Autodesk Inventor part; units mm, degrees
ref_plane "YZ Plane" through (0, 0, 0) normal (1, 0, 0) x (0, 1, 0)
ref_plane "XZ Plane" through (0, 0, 0) normal (0, 1, 0) x (-1, 0, 0)
ref_plane "XY Plane" through (0, 0, 0) normal (0, 0, 1) x (1, 0, 0)
sketch "Sketch1" plane through (0, 0, 0) normal (0, 0, 1) x (1, 0, 0)
  line L0 (45.72, 0) -> (45.72, 60.96)
  line L1 (45.72, 60.96) -> (-45.72, 60.96)
  line L2 (-45.72, 60.96) -> (-45.72, 9.301)
  line L3 (-45.72, 5.08) -> (-50.8, 5.08)
  line L4 (-50.8, 5.08) -> (-50.8, 15.24)
  line L5 (-50.8, 15.24) -> (-45.72, 15.24)
  line L6 (-45.72, 15.24) -> (-45.72, 5.08)
  line L7 (-45.72, 25.4) -> (-50.8, 25.4)
  line L8 (-50.8, 25.4) -> (-50.8, 35.56)
  line L9 (-50.8, 35.56) -> (-45.72, 35.56)
  line L10 (-45.72, 35.56) -> (-45.72, 25.4)
  line L11 (-45.72, 45.72) -> (-50.8, 45.72)
  line L12 (-50.8, 45.72) -> (-50.8, 55.88)
  line L13 (-50.8, 55.88) -> (-45.72, 55.88)
  line L14 (-45.72, 55.88) -> (-45.72, 45.72)
  line L15 (0, 60.96) -> (0, 0) construction
  line L16 (45.72, 60.96) -> (45.72, 0)
  line L17 (45.72, 5.08) -> (50.8, 5.08)
  line L18 (50.8, 5.08) -> (50.8, 15.24)
  line L19 (50.8, 15.24) -> (45.72, 15.24)
  line L20 (45.72, 15.24) -> (45.72, 5.08)
  line L21 (45.72, 25.4) -> (50.8, 25.4)
  line L22 (50.8, 25.4) -> (50.8, 35.56)
  line L23 (50.8, 35.56) -> (45.72, 35.56)
  line L24 (45.72, 35.56) -> (45.72, 25.4)
  line L25 (45.72, 45.72) -> (50.8, 45.72)
  line L26 (50.8, 45.72) -> (50.8, 55.88)
  line L27 (50.8, 55.88) -> (45.72, 55.88)
  line L28 (45.72, 55.88) -> (45.72, 45.72)
  line L29 (-45.72, 5.08) -> (-45.72, 0)
  line L30 (-45.72, 0) -> (45.72, 0)
  line L31 (45.72, 60.96) -> (-45.72, 60.96)
  line L32 (-45.72, 60.96) -> (-45.72, 0)
  line L33 (-45.72, 0) -> (45.72, 0)
  line L34 (45.72, 0) -> (45.72, 60.96)
  dimension "d0" = 91.44
  dimension "d2" = 10.16
  dimension "d3" = 5.08
  dimension "d7" = 20.32
  dimension "d14" = 5.08
  dimension "d15" = 60.96
extrude "Extrusion2" add sketch "Sketch1" along normal blind 5.08
sketch "Sketch5" plane through (0, 0, 5.08) normal (0, 0, 1) x (1, 0, 0)
  line L0 (50.8, 25.4) -> (50.8, 35.56)
  line L1 (50.8, 35.56) -> (45.72, 35.56)
  line L2 (45.72, 35.56) -> (45.72, 45.72)
  line L3 (45.72, 45.72) -> (50.8, 45.72)
  line L4 (50.8, 45.72) -> (50.8, 55.88)
  line L5 (50.8, 55.88) -> (45.72, 55.88)
  line L6 (45.72, 55.88) -> (45.72, 60.96)
  line L7 (45.72, 60.96) -> (-45.72, 60.96)
  line L8 (-45.72, 60.96) -> (-45.72, 55.88)
  line L9 (-45.72, 55.88) -> (-50.8, 55.88)
  line L10 (-50.8, 55.88) -> (-50.8, 45.72)
  line L11 (-50.8, 45.72) -> (-45.72, 45.72)
  line L12 (-45.72, 45.72) -> (-45.72, 35.56)
  line L13 (-45.72, 35.56) -> (-50.8, 35.56)
  line L14 (-50.8, 35.56) -> (-50.8, 25.4)
  line L15 (-50.8, 25.4) -> (-45.72, 25.4)
  line L16 (-45.72, 25.4) -> (-45.72, 15.24)
  line L17 (-45.72, 15.24) -> (-50.8, 15.24)
  line L18 (-50.8, 15.24) -> (-50.8, 5.08)
  line L19 (-50.8, 5.08) -> (-45.72, 5.08)
  line L20 (-45.72, 5.08) -> (-45.72, 0)
  line L21 (-45.72, 0) -> (45.72, 0)
  line L22 (45.72, 0) -> (45.72, 5.08)
  line L23 (45.72, 5.08) -> (50.8, 5.08)
  line L24 (50.8, 5.08) -> (50.8, 15.24)
  line L25 (50.8, 15.24) -> (45.72, 15.24)
  line L26 (45.72, 15.24) -> (45.72, 25.4)
  line L27 (45.72, 25.4) -> (50.8, 25.4)
  line L28 (-24.13, 30.48) -> (24.13, 30.48) construction
  line L29 (-24.13, 21.59) -> (24.13, 21.59)
  line L30 (24.13, 39.37) -> (-24.13, 39.37)
  arc A0 (-24.13, 39.37) -> (-24.13, 21.59) centre (-24.13, 30.48) ccw
  arc A1 (24.13, 21.59) -> (24.13, 39.37) centre (24.13, 30.48) ccw
  line L31 (45.72, 60.96) -> (-45.72, 60.96) construction
  line L32 (0, 60.96) -> (0, 0) construction
  point P0 (0, 30.48)
  dimension "d32" = 48.26
  dimension "d33" = 60.96
  dimension "d34" = 30.48
  dimension "d35" = 8.89
extrude "Extrusion6" cut sketch "Sketch5" against normal blind 25.4 contours A0 L30 A1 L29
sketch "Sketch6" plane through (0, 0, 0) normal (0, 0, -1) x (-1, 0, 0)
  arc A0 (-24.13, 39.37) -> (-24.13, 21.59) centre (-24.13, 30.48) ccw
  line L0 (-24.13, 39.37) -> (24.13, 39.37)
  arc A1 (24.13, 21.59) -> (24.13, 39.37) centre (24.13, 30.48) ccw
  line L1 (24.13, 21.59) -> (-24.13, 21.59)
  line L2 (-50.8, 35.56) -> (-50.8, 25.4)
  line L3 (-50.8, 25.4) -> (-45.72, 25.4)
  line L4 (-45.72, 15.24) -> (-45.72, 25.4)
  line L5 (-50.8, 15.24) -> (-45.72, 15.24)
  line L6 (-50.8, 5.08) -> (-50.8, 15.24)
  line L7 (-45.72, 5.08) -> (-50.8, 5.08)
  line L8 (-45.72, 0) -> (-45.72, 5.08)
  line L9 (45.72, 0) -> (-45.72, 0) construction
  line L10 (45.72, 5.08) -> (45.72, 0)
  line L11 (50.8, 5.08) -> (45.72, 5.08)
  line L12 (50.8, 15.24) -> (50.8, 5.08)
  line L13 (45.72, 15.24) -> (50.8, 15.24)
  line L14 (45.72, 25.4) -> (45.72, 15.24)
  line L15 (45.72, 25.4) -> (50.8, 25.4)
  line L16 (50.8, 25.4) -> (50.8, 35.56)
  line L17 (50.8, 35.56) -> (45.72, 35.56)
  line L18 (45.72, 45.72) -> (45.72, 35.56)
  line L19 (45.72, 45.72) -> (50.8, 45.72)
  line L20 (50.8, 45.72) -> (50.8, 55.88)
  line L21 (50.8, 55.88) -> (45.72, 55.88)
  line L22 (45.72, 60.96) -> (45.72, 55.88)
  line L23 (-45.72, 60.96) -> (45.72, 60.96)
  line L24 (-45.72, 55.88) -> (-45.72, 60.96)
  line L25 (-50.8, 55.88) -> (-45.72, 55.88)
  line L26 (-50.8, 45.72) -> (-50.8, 55.88)
  line L27 (-45.72, 45.72) -> (-50.8, 45.72)
  line L28 (-45.72, 35.56) -> (-45.72, 45.72)
  line L29 (-45.72, 35.56) -> (-50.8, 35.56)
  line L30 (33.02, 30.48) -> (33.02, 60.96)
  line L31 (-45.72, 60.96) -> (45.72, 60.96)
  arc A2 (-24.13, 39.37) -> (-24.13, 21.59) centre (-24.13, 30.48) ccw
  line L32 (-33.02, 30.48) -> (-33.02, 60.96)
  line L33 (-33.02, 60.96) -> (33.02, 60.96)
  arc A3 (24.13, 21.59) -> (24.13, 39.37) centre (24.13, 30.48) ccw
  line L34 (25.8987, 21.7677) -> (0.6317, 16.6382)
  line L35 (-0.6317, 16.6382) -> (-25.8987, 21.7677)
  arc A4 (24.13, 21.59) -> (24.13, 39.37) centre (24.13, 30.48) ccw
  line L36 (0, 21.59) -> (0, 0) construction
  arc A5 (-0.6317, 16.6382) -> (0.6317, 16.6382) centre (0, 19.7498) ccw
  circle A6 centre (24.13, 30.48) radius 8.89
  circle A7 centre (-24.13, 30.48) radius 8.89
  point P0 (0, 16.51)
  dimension "d38" = 5.08
  dimension "d39" = 3.175
extrude "Extrusion7" cut sketch "Sketch6" against normal blind 25.4 contours A0 L32 L23 L30 A1 L0 | A0 L1 A1 L34 A5 L35
equation "\"d7\" = 2 * d2"
equation "\"d34\" = 0.5 * d33"
properties part number "MotorShelf" material "Wood (Birch)"
Geometry: final body of the model. Coordinates: model frame, mm. A direction names the side the tool comes from. Round coordinates to 2 decimals unless told otherwise and drop trailing zeros. Loops run counter-clockwise (first coordinate to the right, second up) from the corner with the lowest first, then second, coordinate; pieces in that order, holes last. Notation, with made-up numbers: (62.25, -27) -> (109.25, -27) arc R8 ccw to (109.25, -21) -> close; hole circle Ø5 at (-11.75, 70). An arc over 180 degrees is marked (long way). Use one line per item in the form item = value. Start each with the question number.
1) Line query: L1, parallel to X at y = 44, z = 4.3; L2, parallel to X at y = 52.5, z = 2.25; L3, parallel to X at y = 3, z = 1.5. Output: solid intervals per line, ascending.
2) Access query for faces 4 (the flat face through (48, 25.4, 3)), 5 (the flat face through (45.72, 3, 3)), 6 (the flat face through (-48, 55.88, 3)), 7 (the flat face through (48, 55.88, 3)). Directions: +Z, -Z, +X, -X, +Y, -Y. A direction counts if a zero-diameter tool reaches every point of the face in a straight line with its end or side. Return the directions, or none.
3) Draft query along X for faces 1 (the flat face through (45.72, 58, 3)), 2 (the flat face through (48, 5.08, 3)), 3 (the flat face through (-13.44, 19.24, 2.5)). Return one class per face: released by +X, released by -X, zero draft, split by the parting line, or undercut.
4) Section A-A on y = 48.5. Output: boundary loops of the cut face in (x, z), then the cut area to 3 significant figures.
5) Section B-B on x = 23.5. Output: boundary loops of the cut face in (y, z), then the cut area to 3 significant figures.
6) Section C-C on y = 23. Output: boundary loops of the cut face in (x, z), then the cut area to 3 significant figures.
7) First-contact query: P1, Ø1.5, axis at x = -49, z = 3, coming from the -Y side; P2, Ø1.5, axis at y = 3.5, z = 1.5, coming from the -X side; P3, Ø1.5, axis at x = -48, z = 2.5, coming from the +Y side. Flat tips, straight axial feed; report the tip coordinate or a pass-through.
8) Section D-D on x = 2. Output: boundary loops of the cut face in (y, z).
Response:
q1.L1 = -45.72 to -33.02, 33.02 to 45.72
q1.L2 = -50.8 to -33.02, 33.02 to 50.8
q1.L3 = -45.72 to 45.72
q2.face_4 = +Z, -Z, +X
q2.face_5 = +Z, -Z, +X, -Y
q2.face_6 = +Z, -Z, -X, +Y
q2.face_7 = +Z, -Z, +X, +Y
q3.face_1 = released by +X
q3.face_2 = zero draft
q3.face_3 = undercut
q4.outline = (-50.8, 0) -> (-33.02, 0) -> (-33.02, 5.08) -> (-50.8, 5.08) -> close; (33.02, 0) -> (50.8, 0) -> (50.8, 5.08) -> (33.02, 5.08) -> close
q4.area = 181 mm^2
q5.outline = (0, 0) -> (21.28, 0) -> (21.28, 5.08) -> (0, 5.08) -> close
q5.area = 108 mm^2
q6.outline = (-45.72, 0) -> (-28.93, 0) -> (-28.93, 5.08) -> (-45.72, 5.08) -> close; (28.93, 0) -> (45.72, 0) -> (45.72, 5.08) -> (28.93, 5.08) -> close
q6.area = 171 mm^2
q7.P1 = 5.08
q7.P2 = -45.72
q7.P3 = 55.88
q8.outline = (0, 0) -> (16.92, 0) -> (16.92, 5.08) -> (0, 5.08) -> close
